Source: three-view drawing plus pictorial views. Frame: mm from the lowest corner of the part. A direction names the side the tool comes from. Give positions to 0.01 mm unless a question says otherwise; leave off trailing zeros. Loops run counter-clockwise (first coordinate to the right, second up) from the corner with the lowest first, then second, coordinate; pieces in that order, holes last.
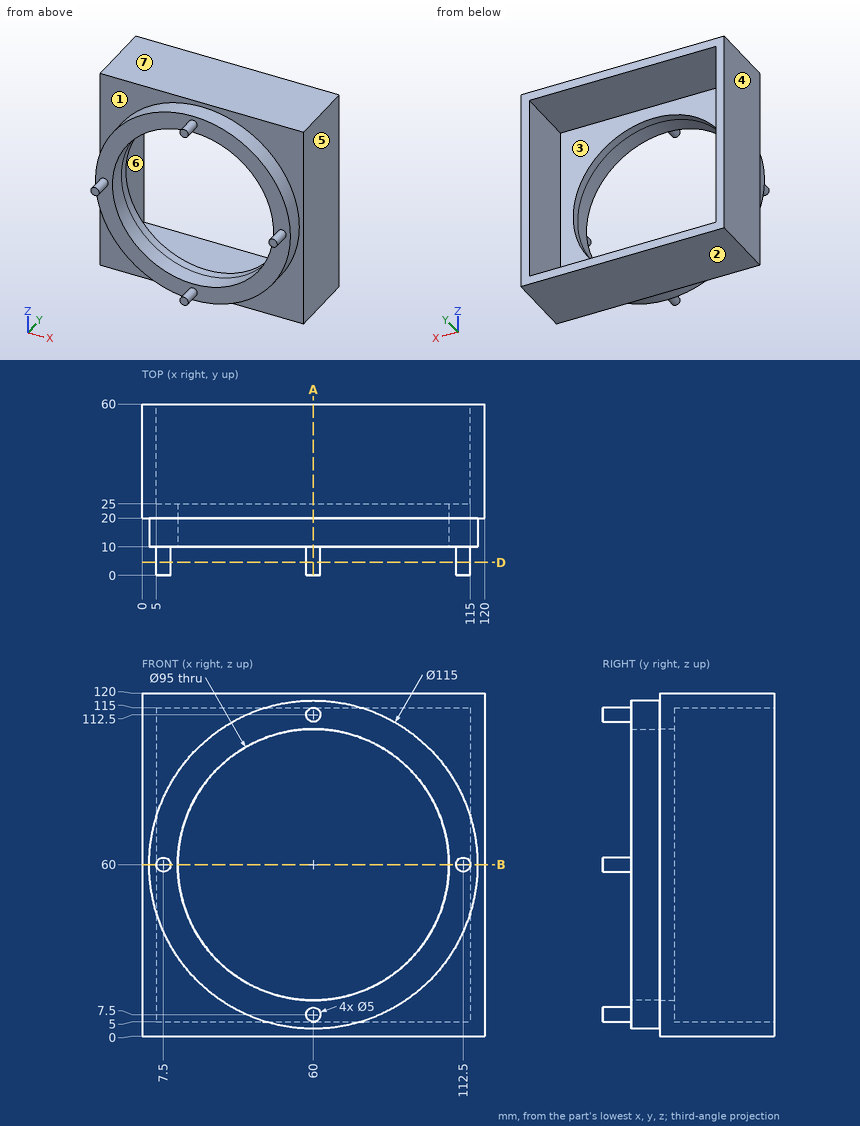
(1) Reachability of the marked faces 1, 2 and 3 from +Z, -Z, +X, -X, +Y, -Y: full face, straight path, thin tool, end or side. Return the list, or none.
Values follow:
face 1: -Y
face 2: -Z, +X, -X, +Y, -Y
face 3: +Y
(2) Cut plane B-B (z = 60). Return the cut outline in (x, y), and give its area (3 significant figures).
Values follow:
outline: (0, 20) - (2.5, 20) - (2.5, 10) - (5, 10) - (5, 0) - (10, 0) - (10, 10) - (12.5, 10) - (12.5, 25) - (5, 25) - (5, 60) - (0, 60) - close; (107.5, 10) - (110, 10) - (110, 0) - (115, 0) - (115, 10) - (117.5, 10) - (117.5, 20) - (120, 20) - (120, 60) - (115, 60) - (115, 25) - (107.5, 25) - close
area: 775 mm2
(3) Cut plane D-D (y = 4.5). Return the cut outline in (x, z).
Values follow:
outline: circle Ø5 at (7.5, 60); circle Ø5 at (60, 7.5); circle Ø5 at (60, 112.5); circle Ø5 at (112.5, 60)
(4) Pin query (flat end, axial travel): pin 1 Ø12 at (x, z) = (39.5, 107.5) entering from +Y. Return the tip coordinate at first contact, or that it passes through.
Values follow:
pin 1: stops at y = 25
(5) Mould query, pull axis X, two halves, no side actions, for the marked faces 4, 5, 6 and 7. Classes: +X half, -X half, draft (parallel to the pull), parting line (faces both ways), or undercut.
Values follow:
face 4: -X half
face 5: +X half
face 6: undercut
face 7: draft
(6) Ray query, probe 1 along Z at (x, y) = (40.5, 51.5); probe 2 along X at (y, z) = (15, 60). Return the intervals inside material, ascending.
Values follow:
probe 1: z = 0 to 5, 115 to 120
probe 2: x = 2.5 to 12.5, 107.5 to 117.5
(7) Cut plane A-A (x = 60). Return the cut outline in (y, z), and give its area (3 significant figures).
Values follow:
outline: (0, 5) - (10, 5) - (10, 2.5) - (20, 2.5) - (20, 0) - (60, 0) - (60, 5) - (25, 5) - (25, 12.5) - (10, 12.5) - (10, 10) - (0, 10) - close; (0, 110) - (10, 110) - (10, 107.5) - (25, 107.5) - (25, 115) - (60, 115) - (60, 120) - (20, 120) - (20, 117.5) - (10, 117.5) - (10, 115) - (0, 115) - close
area: 775 mm2
